Autodesk Inventor part; units mm, degrees
ref_plane "Top Plane for Slope" through (0, 4.5, 0) normal (0, 1, 0) x (-1, 0, 0)
ref_plane "Slope Plane" through (-25.4, 1.5, 25.4) normal (0.0589524, -0.9982608, 0) x (0, 0, -1)
ref_plane "YZ Plane" through (0, 0, 0) normal (1, 0, 0) x (0, 1, 0)
ref_plane "Bottom Plane for Slope" through (0, 1.5, 0) normal (0, 1, 0) x (-1, 0, 0)
sketch "Bottom Plane" plane through (0, 1.5, 0) normal (0, 1, 0) x (-1, 0, 0)
  line L0 (-25.4, 25.4) -> (25.4, 25.4)
  line L1 (25.4, 25.4) -> (25.4, -25.4)
  line L2 (25.4, -25.4) -> (-25.4, -25.4)
  line L3 (-25.4, -25.4) -> (-25.4, 25.4)
  line L4 (-25.4, 25.4) -> (25.4, -25.4) construction
  line L5 (25.4, 25.4) -> (-25.4, -25.4) construction
  point P0 (0, 0)
  dimension "d26" = 50.8
  dimension "d27" = 50.8
ref_plane "Top Plane for Slope" through (0, 4.5, 0) normal (0, 1, 0) x (-1, 0, 0)
sketch "Top Plane" plane through (0, 4.5, 0) normal (0, 1, 0) x (-1, 0, 0)
  line L0 (-25.4, 25.4) -> (25.4, 25.4)
  line L1 (25.4, 25.4) -> (25.4, -25.4)
  line L2 (25.4, -25.4) -> (-25.4, -25.4)
  line L3 (-25.4, -25.4) -> (-25.4, 25.4)
  line L4 (-25.4, 25.4) -> (25.4, -25.4) construction
  line L5 (25.4, 25.4) -> (-25.4, -25.4) construction
  point P0 (0, 0)
  dimension "d28" = 50.8
  dimension "d29" = 50.8
ref_plane "Slope Plane" through (-25.4, 1.5, 25.4) normal (0.0589524, -0.9982608, 0) x (0, 0, -1)
sketch "master" plane through (0, 0, 0) normal (0, 1, 0) x (-1, 0, 0)
  circle A0 centre (0, 0) radius 36
  line L0 (0, 36) -> (0, -36) construction
  line L1 (12, -33.9411) -> (12, 33.9411)
  circle A1 centre (0, 0) radius 10 construction
  line L2 (10, 0) -> (12, 0) construction
  circle A2 centre (-1.7, 0) radius 13.7 construction
  line L3 (-36, 0) -> (12, 0) construction
  circle A3 centre (0, 0) radius 31 construction
  line L4 (7, -35.3129) -> (7, 35.3129) construction
  line L5 (0, 0) -> (-23.1404, -27.5776) construction
  line L6 (0, 0) -> (-23.1404, 27.5776) construction
  circle A4 centre (-1.7, 0) radius 11.7 construction
  line L7 (-1.7, -13.7) -> (-1.7, 13.7) construction
  line L8 (-1.7, -13.7) -> (12, -13.7) construction
  line L9 (-1.7, 13.7) -> (12, 13.7) construction
  point P0 (7, -30.1993)
  point P1 (7, 30.1993)
  point P2 (-19.9264, -23.7474)
  point P3 (-19.9264, 23.7474)
  point P4 (-31, 0)
  point P5 (0, -11.5758)
  point P6 (0, 11.5758)
  point P7 (-13.4, 0)
  dimension "d0" = 72
  dimension "d2" = 20
  dimension "d1" = 2
  dimension "d6" = 27.4
  dimension "d7" = 5
  dimension "d8" = 5
  dimension "d9" = 50
  dimension "d10" = 50
  dimension "d11" = 2
extrude "Main Platform" add sketch "master" along normal blind 5 contours L1 A0 picked at (-3.9243, -1.3458)
sketch "Sketch3" plane through (0, 0, 0) normal (0, -1, 0) x (1, 0, 0)
  circle A0 centre (0, 0) radius 10 construction
  circle A1 centre (0, 0) radius 10
extrude "Main Hole" cut sketch "Sketch3" against normal blind 5
sketch "Sketch4" plane through (0, 0, 0) normal (0, -1, 0) x (1, 0, 0)
  circle A0 centre (1.7, 0) radius 13.7 construction
  circle A1 centre (1.7, 0) radius 13.7
  line L0 (1.7, 13.7) -> (-12, 13.7) construction
  line L1 (1.7, -13.7) -> (-12, -13.7) construction
  line L2 (-12, 13.7) -> (1.7, 13.7)
  line L3 (1.7, 13.7) -> (1.7, -13.7)
  line L4 (1.7, -13.7) -> (-12, -13.7)
  line L5 (-12, -13.7) -> (-12, 13.7)
  point P0 (0, 0)
extrude "Window Recess" cut sketch "Sketch4" against normal blind 1
sketch "Sketch5" plane through (0, 0, 0) normal (0, -1, 0) x (1, 0, 0)
  point P0 (0, 0)
  point P1 (13.4, 0)
hole "Window Removal Holes" at (13.4, 0, 0) direction (0, 1, 0) diameter 1.5 end through all
sketch "Sketch10" plane through (-25.4, 1.5, 25.4) normal (0.0589524, -0.9982608, 0) x (0, 0, -1)
  ellipse E0 centre (25.4, 27.0234) end of major axis (11.7, 27.0234) minor radius 13.6762 (39.1, 27.0234) -> (11.7, 27.0234) ccw construction
  line L0 (11.7, 13.3472) -> (11.7, 27.0234) construction
  line L1 (39.1, 27.0234) -> (39.1, 13.3472) construction
  ellipse E1 centre (25.4, 25.5622) end of major axis (35.4, 25.5622) minor radius 9.9826 construction
  line L2 (59.3411, 13.583) -> (-8.5411, 13.583) construction
  line L3 (39.1, 26.9644) -> (39.1, 13.2883)
  line L4 (39.1, 14.351) -> (11.7, 14.351)
  line L5 (11.7, 14.351) -> (11.7, 35.7061)
  line L6 (11.7, 35.7061) -> (39.1, 35.7061)
  line L7 (39.1, 35.7061) -> (39.1, 14.351)
  point P0 (25.4, 25.2674)
extrude "Slope" add sketch "Sketch10" along normal blind 1
sketch "Sketch14" plane through (0, 0, 0) normal (0, -1, 0) x (1, 0, 0)
  point P0 (0, 0)
  point P1 (-7, 30.1993)
  point P2 (31, 0)
  point P3 (-7, -30.1993)
chamfer "Chamfer1" distance 2 angle 60 1 edges at (-10, 5, 0)
sketch "Sketch17" plane through (-25.4, 1.5, 25.4) normal (0.0589524, -0.9982608, 0) x (0, 0, -1)
  ellipse E0 centre (25.4, 25.4443) end of major axis (25.4, 15.4268) minor radius 10 (15.4, 25.4443) -> (35.4, 25.4443) ccw construction
  ellipse E1 centre (25.4, 26.4797) end of major axis (25.4, 36.6031) minor radius 10.0527 (35.4, 25.4443) -> (15.4, 25.4443) ccw construction
  ellipse E2 centre (25.4, 25.3852) end of major axis (25.4, 15.3678) minor radius 10 construction
  ellipse E3 centre (25.4, 25.4443) end of major axis (35.4, 25.4443) minor radius 9.9826 (15.4, 25.4443) -> (35.4, 25.4443) ccw construction
  line L0 (25.4, 35.4026) -> (32.7708, 19.5959) construction
  line L1 (25.4, 35.4026) -> (18.0292, 19.5959) construction
  line L2 (25.4, 35.4026) -> (25.4, 19.5959) construction
  line L3 (32.7708, 19.5959) -> (18.0292, 19.5959) construction
  line L4 (28.184, 29.4323) -> (22.616, 29.4323) construction
  line L5 (58.9857, 14.0822) -> (-8.1857, 14.0822) construction
  line L6 (-8.1857, 14.0822) -> (-8.1857, 35.4026) construction
  line L7 (-8.1857, 35.4026) -> (58.9857, 35.4026) construction
  line L8 (58.9857, 35.4026) -> (58.9857, 14.0822) construction
  spline S0 degree 5 poles (25.4, 29.4323) (26.7138, 29.432) (28.9448, 27.9113) (31.9512, 21.8517) (32.9232, 20.462) (25.6746, 12.422) (16.6165, 20.5026) (19.1302, 21.7816) (21.8974, 27.8954) (24.0775, 29.4325) (25.4, 29.4323) knots 0 0 0 0 0 0 0.199988 0.334999 0.499228 0.663457 0.798679 1 1 1 1 1 1
  line L9 (30.5619, 24.333) -> (20.2381, 24.333) construction
  line L10 (25.4, 19.5959) -> (25.4, 13.3472) construction
  line L11 (39.1, 13.3472) -> (11.7, 13.3472)
  point P0 (25.4, 25.2674)
  point P1 (25.4, 15.9117)
  point P2 (19.2424, 19.5959)
  dimension "d81" = 25
  dimension "d82" = 25
extrude "Extrusion6" cut sketch "Sketch17" along normal through all
sketch "Sketch15" plane through (0, 5, 0) normal (0, 1, 0) x (1, 0, 0)
  point P0 (0, 0)
  point P1 (31, 0)
  point P2 (-7, -30.1993)
  point P3 (-7, 30.1993)
hole "Top Magnet Holes" at (-7, 5, -30.1993) at (31, 5, 0) at (-7, 5, 30.1993) direction (0, -1, 0) diameter 6.5 depth 0.5
hole "Bottom Magnet Holes" at (-7, 0, 30.1993) at (31, 0, 0) at (-7, 0, -30.1993) direction (0, 1, 0) diameter 6.5 depth 1.5
chamfer "Chamfer7" distance 0.5 angle 45 1 edges at (-12, 2.5, 33.9411)
chamfer "Chamfer8" distance 0.5 angle 45 1 edges at (-12, 2.5, -33.9411)
chamfer "Chamfer9" distance 0.5 angle 45 1 edges at (-12, 5, -19.7735)
chamfer "Chamfer10" distance 0.5 angle 45 1 edges at (-12, 5, 19.7735)
chamfer "Chamfer11" distance 0.5 angle 45 1 edges at (-12, 0, 23.5706)
chamfer "Chamfer12" distance 0.5 angle 45 1 edges at (-12, 0, -23.5706)
chamfer "Chamfer13" distance 0.5 angle 45 1 edges at (36, 5, 0)
chamfer "Chamfer14" distance 0.5 angle 45 1 edges at (36, 0, 0)
chamfer "Chamfer15" distance 0.5 angle 45 1 edges at (-7, 5, -33.4493)
chamfer "Chamfer16" distance 0.5 angle 45 1 edges at (31, 5, -3.25)
chamfer "Chamfer17" distance 0.5 angle 45 1 edges at (-7, 5, 26.9493)
chamfer "Chamfer18" distance 0.5 angle 45 1 edges at (-7, 0, 33.4493)
chamfer "Chamfer19" distance 0.5 angle 45 1 edges at (31, 0, 3.25)
chamfer "Chamfer20" distance 0.5 angle 45 1 edges at (-7, 0, -26.9493)
properties part number "holder"
Check sheet for the modelled part. Datum: model origin and axes. Units: mm. A direction names the side the tool comes from. Round coordinates to 2 decimals unless told otherwise and drop trailing zeros. Write item = value, one per line. Start each with the question number.
1. Release check for a two-part mould opening along X. For faces 4 (the cylindrical face through (34.173, 1.007, 0.705)), 5 (the flat face through (-12, 2, 0)) record: pulls with the +X half, pulls with the -X half, needs draft (parallel to the pull), parting line crosses it, or undercut.
2. Tool access check on faces 1 (the flat face through (31, 1.5, 0)), 2 (the flat face through (-7, 4.5, 30)), 3 (the cylindrical face through (15.397, 0.493, -0.301)). Record the directions out of +Z, -Z, +X, -X, +Y, -Y that give a thin tool (end or side, any length) a straight path to the whole face; none if there is none.
3. Section check A-A, the plane z = 0. State how many separate pieces and enclosed holes the cut face has, then the cut area to 3 significant figures.
4. Scan lines: line 1 (X direction, y = 0.85, z = 0); line 2 (X direction, y = 1.25, z = 0); line 3 (Z direction, x = -7, y = 4.55). Record each from-to range of solid material in increasing order. Write a range as [from, to].
5. Gauge pin test, flat ends, axial feed: pin 1 (2 mm diameter, centred on x = -7, z = 29.5, fed in from -Y); pin 2 (2 mm diameter, centred on x = 15, y = 0.5, fed in from -Z); pin 3 (3 mm diameter, centred on x = 5.5, y = 3, fed in from -Z). Record the tip position at first contact, or that the pin passes through.
Results found:
q1.face_4 = undercut
q1.face_5 = pulls with the -X half
q2.face_1 = -Y
q2.face_2 = +Y
q2.face_3 = -X, -Y
q3.separate_pieces = 3
q3.enclosed_holes = 0
q3.area = 114 mm^2
q4.line_1 = [15.4, 27.75], [34.25, 36]
q4.line_2 = [-12, -10], [10, 12.65], [14.15, 27.75], [34.25, 36]
q4.line_3 = [-35.26, -33.5], [-26.9, -10.58], [10.58, 26.9], [33.5, 35.26]
q5.pin_1 = 1.5
q5.pin_2 = -33.17
q5.pin_3 = -35.78
